from build123d import *

# Parameters (mm, degrees)
SKETCH2_R           = 1
FILLET1_R           = 1
SKETCH3_R           = 2
BOSS_EXTRUDE1_DEPTH = 2.5


with BuildPart() as part:
    # Sweep2: sweep along a path in Sketch1
    with BuildLine(Plane(origin=(0, 0, 0), x_dir=(1, 0, 0), z_dir=(0, 1, 0))) as sweep2_path:
        Line((0, -17), (0, -3))
        ThreePointArc((0, -3), (0.878679656, -0.878679656), (3, 0))
        Line((3, 0), (17, 0))
    # Sketch2 → Sweep2 (sweep)
    with BuildSketch(Plane(origin=(17, 0, 0), x_dir=(0, 0, -1), z_dir=(1, 0, 0))):
        Circle(SKETCH2_R)
    sweep(path=sweep2_path.line)

    # Fillet1
    fillet1_edges = [part.edges().sort_by_distance(p)[0] for p in [
        (1, 0, 17),
    ]]
    fillet(fillet1_edges, radius=FILLET1_R)

    # Sketch3 → Boss-Extrude1 (add)
    with BuildSketch(Plane(origin=(17, 0, 0), x_dir=(0, 0, -1), z_dir=(1, 0, 0))):
        Circle(SKETCH3_R)
    extrude(amount=BOSS_EXTRUDE1_DEPTH)


solid = part.part
CAD build for the part. Positions are in the model's coordinates, mm. Give positions to 0.01 mm unless a question says otherwise; leave off trailing zeros. Loops run counter-clockwise (first coordinate to the right, second up) from the corner with the lowest first, then second, coordinate; pieces in that order, holes last. Notation, with made-up numbers: M -31.75,82.5 L 11.25,82.5 A20 cw 11.25,107.5 Z; hole C 46,37.5 d9. An arc over 180 degrees is marked long. Answer in a Markdown table with one row per item. Add a question column.
Item 1: Probe probe 1 along Y at (x, z) = (0, 8); probe 2 along Z at (x, y) = (18.75, -0.1). List the from-to ranges inside material, lowest first.
Item 2: Mould opens along X. For faces 1 (the face through (10, -1, 0)), 2 (the face through (17, -1, -1)), 3 (the face through (19.5, 0, 0)), 4 (the face through (18, -2, 0)) say: +X half, -X half, draft (parallel to the pull), parting line (faces both ways), or undercut.
Item 3: Band-saw the part on B-B on z = 7.5. Give the cut face in (x, y), then the cut area to 3 significant figures.
Item 4: Band-saw the part on A-A on y = 0. Give the cut face in (x, z), then the cut area to 3 significant figures.
Item 5: Drop flat-ended pins along their axis: P1, Ø2, axis at y = -0.5, z = 1, coming from the -X side; P2, Ø8, axis at x = 3, z = 13, coming from the -Y side. Give the stop position or say it passes through.
Item 6: Band-saw the part on D-D on y = 1.7. Give the cut face in (x, z).
Reply:
| question | item | result |
|---|---|---|
| 1 | probe 1 | y = -1 to 1 |
| 1 | probe 2 | z = -2 to 2 |
| 2 | face 1 | undercut |
| 2 | face 2 | undercut |
| 2 | face 3 | +X half |
| 2 | face 4 | draft |
| 3 | outline | C 0,0 d2 |
| 3 | area | 3.14 mm^2 |
| 4 | outline | M -1,3 A4 ccw 3,-1 L 17,-1 L 17,-2 L 19.5,-2 L 19.5,2 L 17,2 L 17,1 L 3,1 A2 cw 1,3 L 1,16 A1 ccw -1,16 Z |
| 4 | area | 75.0 mm^2 |
| 5 | P1 | stops at x = -0.85 |
| 5 | P2 | stops at y = -1 |
| 6 | outline | M 17,-1.05 L 19.5,-1.05 L 19.5,1.05 L 17,1.05 Z |
